from build123d import *

# Parameters (mm, degrees)
SKETCH1_R          = 35
EXTRUDE1_DEPTH     = 25
SKETCH2_R          = 12.5
CUT_EXTRUDE1_DEPTH = 56.452682532
SKETCH3_W          = 10
SKETCH3_H          = 15.734862576
CUT_EXTRUDE2_DEPTH = 15
FILLET1_R          = 5
SKETCH4_R          = 22.5
CUT_EXTRUDE4_DEPTH = 5
SKETCH5_R          = 4
SIDE_HOLE_DEPTH    = 56.452682595


with BuildPart() as part:
    # Sketch1 → Extrude1 (new body)
    with BuildSketch(Plane.XY):
        Circle(SKETCH1_R)
    extrude(amount=EXTRUDE1_DEPTH)

    # Sketch2 → Cut-Extrude1 (cut, through all)
    with BuildSketch(Plane.XY.offset(25)):
        Circle(SKETCH2_R)
    extrude(amount=-CUT_EXTRUDE1_DEPTH, mode=Mode.SUBTRACT)

    # Sketch3 → Cut-Extrude2 (cut)
    with BuildSketch(Plane.XY.offset(25)):
        with Locations((0, 32.867431288)):
            Rectangle(SKETCH3_W, SKETCH3_H)
    extrude(amount=-CUT_EXTRUDE2_DEPTH, mode=Mode.SUBTRACT)

    # Fillet1
    # the kernel refuses this fillet: 5 mm, written as the material it adds along each edge
    with BuildSketch(Plane(origin=(-5, 12.5, 10), x_dir=(0, 0, 1), z_dir=(0, 1, 0))) as fillet1_piece_1_section:
        with BuildLine():
            CenterArc((FILLET1_R, FILLET1_R), FILLET1_R, 180, 90)
            Line((0, FILLET1_R), (0, 0))
            Line((0, 0), (FILLET1_R, 0))
        make_face()
    fillet1_piece_1 = extrude(amount=34.641016151, mode=Mode.PRIVATE)
    fillet1_piece_1 = fillet1_piece_1 & Plane(origin=(0, 0, 10), x_dir=(1, 0, 0), z_dir=(0, 0, -1)) * Cylinder(35, 90, mode=Mode.PRIVATE)
    with BuildSketch(Plane(origin=(5, 47.141016151, 10), x_dir=(-1, 0, 0), z_dir=(0, -1, 0))) as fillet1_piece_2_section:
        with BuildLine():
            CenterArc((FILLET1_R, -FILLET1_R), FILLET1_R, 90, 90)
            Line((0, -FILLET1_R), (0, 0))
            Line((0, 0), (FILLET1_R, 0))
        make_face()
    fillet1_piece_2 = extrude(amount=34.641016151, mode=Mode.PRIVATE)
    fillet1_piece_2 = fillet1_piece_2 & Plane(origin=(0, 0, 10), x_dir=(1, 0, 0), z_dir=(0, 0, -1)) * Cylinder(35, 90, mode=Mode.PRIVATE)
    add([fillet1_piece_1, fillet1_piece_2])

    # Sketch4 → Cut-Extrude4 (cut)
    with BuildSketch(Plane(origin=(0, 0, 0), x_dir=(-1, 0, 0), z_dir=(0, 0, -1))):
        Circle(SKETCH4_R)
    extrude(amount=-CUT_EXTRUDE4_DEPTH, mode=Mode.SUBTRACT)

    # Sketch5 → Side hole (cut, through all)
    with BuildSketch(Plane(origin=(0, 0, 0), x_dir=(0, 0, -1), z_dir=(1, 0, 0))):
        with Locations((-12.5, -0.089745962)):
            Circle(SKETCH5_R)
    extrude(amount=-SIDE_HOLE_DEPTH, mode=Mode.SUBTRACT)


solid = part.part
Verification items for the finished model (mm, model axes). A direction names the side the tool comes from. Coordinates: 2 decimals unless noted, no trailing zeros. Order: outer loops, then holes, each group sorted by start corner. A loop starts at its lowest first (then second) coordinate and runs counter-clockwise, first axis right, second up. Notation, with made-up numbers: (83, -38) -> (104, -38) arc R32 cw to (104, -7) -> close; hole circle Ø3 at (78, 46.5). An arc over 180 degrees is marked (long way). Use CSV: the item, a comma, the result in double quotes. Start each with the question number.
Q1. Section check B-B, the plane x = 7. Record the cut outline in (y, z).
Q2. Section check C-C, the plane z = 2. Record the cut outline in (x, y).
Q3. Section check D-D, the plane y = 11. Record the cut outline in (x, z), and give its area (3 significant figures).
Q4. Thickness scan on line 1 along Y through (x, z) = (0, 3.25); line 2 along Y through (x, z) = (0, 16.75); line 3 along Z through (x, y) = (1.5, 17). Record the ranges inside material, lowest first.
Q5. Depth check by flat-ended pin: P1, Ø5, axis at y = 9.5, z = 6.5, coming from the +X side; P2, Ø2, axis at x = 4.5, z = 16, coming from the -Y side; P3, Ø1.5, axis at x = 9.5, y = 16, coming from the -Z side; P4, Ø2, axis at x = 24.5, y = 16.5, coming from the -Z side. Enter the tip coordinate at first touch or a pass-through.
Q6. Section check A-A, the plane x = -16.5. Record the cut outline in (y, z), and give its area (3 significant figures).
Q7. Draft check along Y on faces 1 (the cylindrical face through (11.923, 3.755, 15.14)), 2 (the flat face through (0, 25, 18)), 3 (the cylindrical face through (-10.382, -19.961, 2.465)), 4 (the flat face through (-5, 30, 20)). Enter one of: +Y half, -Y half, draft (parallel to the pull), parting line (faces both ways), or undercut.
Q8. Tool access check on faces 5 (the cylindrical face through (-23.245, 0.086, 16.496)), 6 (the flat face through (5, 30, 20)), 7 (the flat face through (-10, -10, 5)). Record the directions out of +Z, -Z, +X, -X, +Y, -Y that give a thin tool (end or side, any length) a straight path to the whole face; none if there is none.
Returned:
1,outline,"(-34.29, 0) -> (-21.38, 0) -> (-21.38, 5) -> (-10.36, 5) -> (-10.36, 25) -> (-34.29, 25) -> close; (10.36, 5) -> (21.38, 5) -> (21.38, 0) -> (34.29, 0) -> (34.29, 25) -> (10.36, 25) -> close"
2,outline,"circle Ø70 at (0, 0); hole circle Ø45 at (0, 0)"
3,outline,"(-33.23, 0) -> (-19.63, 0) -> (-19.63, 5) -> (-5.94, 5) -> (-5.94, 25) -> (-33.23, 25) -> close; (5.94, 5) -> (19.63, 5) -> (19.63, 0) -> (33.23, 0) -> (33.23, 25) -> (5.94, 25) -> close"
3,area,"1,230 mm^2"
4,line 1,"y = -35 to -22.5, 22.5 to 35"
4,line 2,"y = -35 to -12.5, 12.5 to 25"
4,line 3,"z = 5 to 25"
5,P1,"stops at x = 34.29"
5,P2,"stops at y = -34.82"
5,P3,"stops at z = 5"
5,P4,"stops at z = 0"
6,outline,"(-30.87, 0) -> (-15.3, 0) -> (-15.3, 5) -> (15.3, 5) -> (15.3, 0) -> (30.87, 0) -> (30.87, 25) -> (-30.87, 25) -> close; hole circle Ø8 at (-0.09, 12.5)"
6,area,"1,340 mm^2"
7,face 1,"undercut"
7,face 2,"+Y half"
7,face 3,"undercut"
7,face 4,"draft"
8,face 5,"-X"
8,face 6,"+Z, +Y"
8,face 7,"-Z"
